Geometry check sheet. Reference: drawing and pictorial views, mm from the part's lowest x, y, z. A direction names the side the tool comes from. Round coordinates to 2 decimals unless told otherwise and drop trailing zeros. Order: outer loops, then holes, each group sorted by start corner. A loop starts at its lowest first (then second) coordinate and runs counter-clockwise, first axis right, second up.
(1) Draft check along X on the marked faces 3, 4, 5 and 6. Enter one of: pulls with the +X half, pulls with the -X half, needs draft (parallel to the pull), parting line crosses it, or undercut.
(2) Thickness scan on L1, parallel to Z at x = 4.75, y = 1.85; L2, parallel to X at y = 1.8, z = 7.25 (1 decimal); L3, parallel to X at y = 1.4, z = 3 (1 decimal). Record the ranges inside material, lowest first.
(3) Cross-section at A-A on x = 2.25. Enter the section's corners in (y, z).
(4) Cross-section at C-C on y = 1.1. Enter the section's corners in (x, z).
(5) Cross-section at B-B on z = 3.75. Enter the section's corners in (x, y).
(6) Set-up check for the marked faces 1 and 2: record each of +Z, -Z, +X, -X, +Y, -Y from which the full face is reachable in a straight line by a thin tool's end or side.
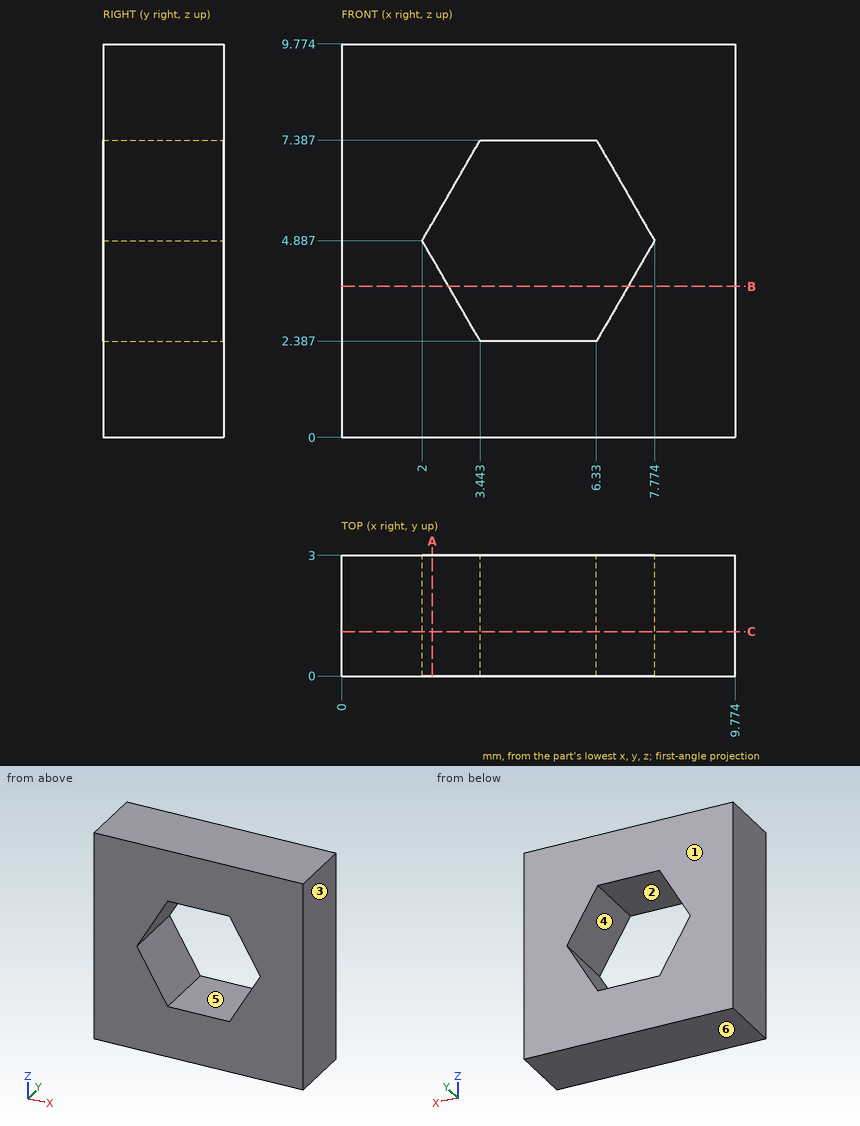
Found:
1. face 3: pulls with the +X half
1. face 4: undercut
1. face 5: undercut
1. face 6: needs draft
2. L1: z = 0 to 2.39, 7.39 to 9.77
2. L2: x = 0 to 3.4, 6.4 to 9.8
2. L3: x = 0 to 3.1, 6.7 to 9.8
3. outline: (0, 0) - (3, 0) - (3, 4.45) - (0, 4.45) - close; (0, 5.32) - (3, 5.32) - (3, 9.77) - (0, 9.77) - close
4. outline: (0, 0) - (9.77, 0) - (9.77, 9.77) - (0, 9.77) - close; hole (2, 4.89) - (3.44, 2.39) - (6.33, 2.39) - (7.77, 4.89) - (6.33, 7.39) - (3.44, 7.39) - close
5. outline: (0, 0) - (2.66, 0) - (2.66, 3) - (0, 3) - close; (7.12, 0) - (9.77, 0) - (9.77, 3) - (7.12, 3) - close
6. face 1: +Z, -Z, +X, -X, +Y
6. face 2: +Y, -Y
